For this review, take the finished solid that the model builds, in its own axes (mm). A direction names the side the tool comes from. Round coordinates to 2 decimals unless told otherwise and drop trailing zeros. Write each loop counter-clockwise with the first axis right and the second up, starting at its lowest first coordinate (ties: lowest second). Pieces come first, ordered by that corner, then holes. Notation, with made-up numbers: M 27,89 L 81,89 A22 ccw 81,107 Z; hole C -17,-15 d8. An arc over 180 degrees is marked long. One line per question, with ' | ' between items.
Autodesk Inventor part; units mm, degrees
ref_plane "YZ Plane" through (0, 0, 0) normal (1, 0, 0) x (0, 1, 0)
ref_plane "XZ Plane" through (0, 0, 0) normal (0, 1, 0) x (-1, 0, 0)
ref_plane "XY Plane" through (0, 0, 0) normal (0, 0, 1) x (1, 0, 0)
sketch "Sketch1" plane through (0, 0, 0) normal (0, 0, 1) x (1, 0, 0)
  line L0 (-15.5, 60) -> (15.5, 60)
  line L1 (15.5, 60) -> (15.5, -57)
  line L2 (-15.5, -57) -> (-15.5, 60)
  line L3 (-15.5, 60) -> (15.5, -60) construction
  line L4 (15.5, 60) -> (-15.5, -60) construction
  line L5 (15.5, -57) -> (6.2, -57)
  line L6 (6.2, -57) -> (6.2, -60)
  line L7 (2.65, -60) -> (2.65, -57)
  line L8 (2.65, -57) -> (1.5, -57)
  line L9 (1.5, -57) -> (1.5, -55)
  line L10 (1.5, -55) -> (2.65, -55)
  line L11 (2.65, -55) -> (2.65, -52.6)
  line L12 (2.65, -52.6) -> (1.5, -52.6)
  line L13 (1.5, -52.6) -> (1.5, -52)
  line L14 (1.5, -52) -> (-1.5, -52)
  line L15 (-1.5, -52) -> (-1.5, -52.6)
  line L16 (-1.5, -52.6) -> (-2.65, -52.6)
  line L17 (-2.65, -52.6) -> (-2.65, -55)
  line L18 (-2.65, -55) -> (-1.5, -55)
  line L19 (-1.5, -57) -> (-2.65, -57)
  line L20 (-1.5, -55) -> (-1.5, -57)
  line L21 (-2.65, -57) -> (-2.65, -60)
  line L22 (-15.5, -57) -> (-6.2, -57)
  line L23 (-6.2, -57) -> (-6.2, -60)
  line L24 (0, -51.179) -> (0, -61.7681) construction
  line L25 (6.2, -60) -> (2.65, -60)
  line L26 (-2.65, -60) -> (-6.2, -60)
  line L27 (-24.2882, 0) -> (26.7754, 0) construction
  circle A0 centre (0, -15.4294) radius 3.9
  circle A1 centre (0, 33.4294) radius 3.9
  point P0 (0, 0)
  dimension "d0" = 31
  dimension "d4" = 3
  dimension "d6" = 3
  dimension "d7" = 2.4
  dimension "d10" = 5.3
  dimension "d11" = 8
  dimension "d12" = 5
  dimension "d13" = 12.4
  dimension "d14" = 7.8
  dimension "d15" = 44.5706
  dimension "d16" = 7.8
  dimension "d17" = 93.4294
extrude "Extrusion1" add sketch "Sketch1" along normal blind 3
equation "\"d13\" = 0.4 * d0"
properties part number "Y-Shaft-Holder-Front"
Item 1: Take a section at B-B (y = 35). Write out the cut boundary in (x, z), then the cut area to 3 significant figures.
Results:
outline: M -15.5,0 L -3.57,0 L -3.57,3 L -15.5,3 Z; M 3.57,0 L 15.5,0 L 15.5,3 L 3.57,3 Z | area: 71.6 mm2
Item 2: To check wall thickness, follow line 1 along Y through (x, z) = (0, 1.3); line 2 along Y through (x, z) = (1, 2.65); line 3 along Y through (x, z) = (-2.5, 2.55). State the ranges of each line that lie inside material, in increasing order. Write a range as from..to.
Results:
line 1: -52..-19.33, -11.53..29.53, 37.33..60 | line 2: -52..-19.2, -11.66..29.66, 37.2..60 | line 3: -57..-55, -52.6..-18.42, -12.44..30.44, 36.42..60
Item 3: Take a section at C-C (z = 1.5). Write out the cut boundary in (x, y), then the cut area to 3 significant figures.
Results:
outline: M -15.5,-57 L -6.2,-57 L -6.2,-60 L -2.65,-60 L -2.65,-57 L -1.5,-57 L -1.5,-55 L -2.65,-55 L -2.65,-52.6 L -1.5,-52.6 L -1.5,-52 L 1.5,-52 L 1.5,-52.6 L 2.65,-52.6 L 2.65,-55 L 1.5,-55 L 1.5,-57 L 2.65,-57 L 2.65,-60 L 6.2,-60 L 6.2,-57 L 15.5,-57 L 15.5,60 L -15.5,60 Z; hole C 0,-15.43 d7.8; hole C 0,33.43 d7.8 | area: 3,530 mm2
Item 4: Take a section at A-A (x = 0). Write out the cut boundary in (y, z).
Results:
outline: M -52,0 L -19.33,0 L -19.33,3 L -52,3 Z; M -11.53,0 L 29.53,0 L 29.53,3 L -11.53,3 Z; M 37.33,0 L 60,0 L 60,3 L 37.33,3 Z
Item 5: Machinability: for faces 1 (the face through (11, -57, 1)), 2 (the face through (-2.65, -58, 1)), 3 (the face through (-6.2, -58, 1)), which of the approach directions +Z, -Z, +X, -X, +Y, -Y give a long, thin tool a straight path to every point of the face, cutting with its end or side? Answer none if there is none.
Results:
face 1: +Z, -Z, +X, -Y | face 2: +Z, -Z, -Y | face 3: +Z, -Z, -X, -Y
Item 6: Insertion check: pin 1 Ø0.9 at (x, z) = (11, 2) entering from -Y; pin 2 Ø0.9 at (y, z) = (-58.5, 1) entering from -X; pin 3 Ø6 at (x, y) = (0, -15.43) entering from -Z; pin 4 Ø1.5 at (y, z) = (-58, 1) entering from +X. Each pin has a flat end and moves straight along its axis. Give the tip position at first contact, or say it passes through.
Results:
pin 1: y = -57 | pin 2: x = -6.2 | pin 3: through | pin 4: x = 6.2
Item 7: Mouldability with a two-part tool opening along X and no side actions: class faces 4 (the face through (-1.5, -56, 1)), 5 (the face through (-15.5, 1, 1)), 6 (the face through (15.5, 2, 1)), 7 (the face through (1.8, 36.89, 1.48)) as +X half, -X half, draft (parallel to the pull), parting line (faces both ways), or undercut.
Results:
face 4: undercut | face 5: -X half | face 6: +X half | face 7: undercut
Item 8: Take a section at D-D (x = 8.5). Write out the cut boundary in (y, z), then the cut area to 3 significant figures.
Results:
outline: M -57,0 L 60,0 L 60,3 L -57,3 Z | area: 351 mm2
